Here's how the part is built. I have some questions about the finished solid (model axes, mm). Face numbers are marked on the shaded views. Round coordinates to 2 decimals unless told otherwise and drop trailing zeros. Order: outer loops, then holes, each group sorted by start corner. A loop starts at its lowest first (then second) coordinate and runs counter-clockwise, first axis right, second up. Notation, with made-up numbers: (57, 27.5) - (93, 27.5) arc R15 ccw to (93, 54.5) - close; hole circle Ø1 at (-27, 31.25). An arc over 180 degrees is marked (long way). One line per item, written item: value.
from build123d import *

# Parameters (mm, degrees)
SKETCH_1_W          = 99.97480061
SKETCH_1_H          = 51.97470409
EXTRUDE_1_DEPTH     = 5
SKETCH_2_W          = 96.97480061
SKETCH_2_H          = 48.730863602
CUT_EXTRUDE_1_DEPTH = 3
SKETCH_3_R          = 1.1
CUT_EXTRUDE_2_DEPTH = 1437.467063218
FILLET_1_R          = 3
FILLET_2_R          = 2
SKETCH_4_R          = 2.1
CUT_EXTRUDE_3_DEPTH = 1


with BuildPart() as part:
    # 草图1 → 凸台-拉伸1 (new body)
    with BuildSketch(Plane.XY.offset(1066.885602923)):
        with Locations((934.401162421, 1020.144466268)):
            Rectangle(SKETCH_1_W, SKETCH_1_H)
    extrude(amount=EXTRUDE_1_DEPTH)

    # 草图2 → 切除-拉伸1 (cut)
    with BuildSketch(Plane(origin=(0, 0, 1066.885602923), x_dir=(-1, 0, 0), z_dir=(0, 0, -1))):
        with Locations((-934.401162421, 1020.022546024)):
            Rectangle(SKETCH_2_W, SKETCH_2_H)
    extrude(amount=-CUT_EXTRUDE_1_DEPTH, mode=Mode.SUBTRACT)

    # 草图3 → 切除-拉伸2 (cut, through all)
    with BuildSketch(Plane.XY.offset(1071.885602923)):
        with Locations((972.388562726, 1041.631818313)):
            Circle(SKETCH_3_R)
        with Locations((972.388562726, 998.657114223)):
            Circle(SKETCH_3_R)
        with Locations((920.413762116, 998.657114223)):
            Circle(SKETCH_3_R)
        with Locations((920.413762116, 1041.631818313)):
            Circle(SKETCH_3_R)
    extrude(amount=-CUT_EXTRUDE_2_DEPTH, mode=Mode.SUBTRACT)

    # 圆角1
    fillet_1_edges = [part.edges().sort_by_distance(p)[0] for p in [
        (884.413762116, 1046.131818313, 1069.385602923),
        (984.388562726, 1046.131818313, 1069.385602923),
        (984.388562726, 994.157114223, 1069.385602923),
        (884.413762116, 994.157114223, 1069.385602923),
    ]]
    fillet(fillet_1_edges, radius=FILLET_1_R)

    # 圆角2
    fillet_2_edges = [part.edges().sort_by_distance(p)[0] for p in [
        (982.888562726, 995.657114223, 1068.385602923),
        (982.888562726, 1044.387977825, 1068.385602923),
        (885.913762116, 1044.387977825, 1068.385602923),
        (885.913762116, 995.657114223, 1068.385602923),
    ]]
    fillet(fillet_2_edges, radius=FILLET_2_R)

    # 草图4 → 切除-拉伸3 (cut)
    with BuildSketch(Plane.XY.offset(1071.885602923)):
        with Locations((920.299535548, 1041.644508178)):
            Circle(SKETCH_4_R)
        with Locations((972.388562726, 1041.631818313)):
            Circle(SKETCH_4_R)
        with Locations((972.388562726, 998.657114223)):
            Circle(SKETCH_4_R)
        with Locations((920.413762116, 998.657114223)):
            Circle(SKETCH_4_R)
    extrude(amount=-CUT_EXTRUDE_3_DEPTH, mode=Mode.SUBTRACT)


solid = part.part
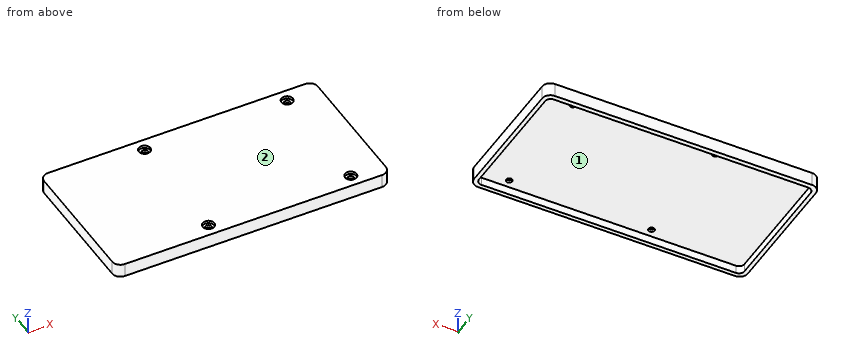
Q1. If we section it at A-A, the plane z = 1068.45: Please give me the cut outline in (x, y), then the cut area to 3 significant figures.
Results list:
outline: (884.41, 997.16) arc R3 ccw to (887.41, 994.16) - (981.39, 994.16) arc R3 ccw to (984.39, 997.16) - (984.39, 1043.13) arc R3 ccw to (981.39, 1046.13) - (887.41, 1046.13) arc R3 ccw to (884.41, 1043.13) - close; hole (885.91, 997.66) arc R2 ccw to (887.91, 995.66) - (980.89, 995.66) arc R2 ccw to (982.89, 997.66) - (982.89, 1042.39) arc R2 ccw to (980.89, 1044.39) - (887.91, 1044.39) arc R2 ccw to (885.91, 1042.39) - close
area: 466 mm²
Q2. If I drill on line 1 along X through (y, z) = (1001.5, 1067.2); line 2 along Y through (x, z) = (953, 1067.25); line 3 along Z through (x, y) = (916.5, 1015), over which ranges is the centre line in solid material (lowest first)?
Results list:
line 1: 884.41 to 885.91, 982.89 to 984.39
line 2: 994.16 to 995.66, 1044.39 to 1046.13
line 3: 1069.89 to 1071.89
Q3. Will these pins go through, and if not, where does the flat tip stop? pin 1 (14.5 mm diameter, centred on x = 910.5, y = 1020.5, fed in from -Z); pin 2 (3.5 mm diameter, centred on x = 972.5, y = 1041.5, fed in from +Z).
Results list:
pin 1: z = 1069.89
pin 2: z = 1070.89
Q4. If we section it at C-C, the plane x = 962.5: Please give me the cut outline in (y, z), then the cut area to 3 significant figures.
Results list:
outline: (994.16, 1066.89) - (995.66, 1066.89) - (995.66, 1069.89) - (1044.39, 1069.89) - (1044.39, 1066.89) - (1046.13, 1066.89) - (1046.13, 1071.89) - (994.16, 1071.89) - close
area: 114 mm²
Q5. If we section it at B-B, the plane y = 1002: Please give me the cut outline in (x, z).
Results list:
outline: (884.41, 1066.89) - (885.91, 1066.89) - (885.91, 1069.89) - (982.89, 1069.89) - (982.89, 1066.89) - (984.39, 1066.89) - (984.39, 1071.89) - (884.41, 1071.89) - close
Q6. We'd pull the mould along X, two halves only. Please class the marked faces 1 and 2: released by +X, released by -X, zero draft, split by the parting line, or undercut.
Results list:
face 1: undercut
face 2: zero draft
